Geometry: final body of the model. Coordinates: model frame, mm. A direction names the side the tool comes from. Coordinates: 2 decimals unless noted, no trailing zeros. Order: outer loops, then holes, each group sorted by start corner. A loop starts at its lowest first (then second) coordinate and runs counter-clockwise, first axis right, second up. Notation, with made-up numbers: M -4.75,36 L 12.25,36 A31 cw 12.25,70 Z; hole C 35,3 d6. An arc over 180 degrees is marked long. Use CSV: the item, a comma, the result in double quotes. Start each with the question number.
Q1. Section query C-C, the plane z = 1.6. Output: boundary loops of the cut face in (x, y), and give its area (3 significant figures).
Q2. First-contact query: P1, Ø1, axis at y = -1.5, z = 0.5, coming from the +X side. Flat tip, straight axial feed; report the tip coordinate or a pass-through.
Q3. Access query for faces 3 (the face through (-1, 2, 1.785)), 4 (the face through (2.5, 1.917, 0.859)). Directions: +Z, -Z, +X, -X, +Y, -Y. A direction counts if a zero-diameter tool reaches every point of the face in a straight line with its end or side. Return the directions, or none.
Q4. Section query D-D, the plane z = 0.5. Output: boundary loops of the cut face in (x, y), and give its area (3 significant figures).
Q5. Ray query, probe 1 along Y at (x, z) = (0, 1.55); probe 2 along X at (y, z) = (0, 0.9). Return the intervals inside material, ascending.
Q6. Mould query, pull axis X, two halves, no side actions, for faces 1 (the face through (-2.604, -0.82, 1.695)), 2 (the face through (0.748, 0.976, 1.122)). Classes: +X half, -X half, draft (parallel to the pull), parting line (faces both ways), or undercut.
Autodesk Inventor part; units mm, degrees
ref_plane "YZ Plane" through (0, 0, 0) normal (1, 0, 0) x (0, 1, 0)
ref_plane "XZ Plane" through (0, 0, 0) normal (0, 1, 0) x (-1, 0, 0)
ref_plane "XY Plane" through (0, 0, 0) normal (0, 0, 1) x (1, 0, 0)
sketch "Sketch2" plane through (0, 0, 0) normal (0, 1, 0) x (-1, 0, 0)
  line L0 (0, 0) -> (0, 2.27)
  line L1 (0, 0) -> (3.15, 0)
  line L2 (3.15, 0) -> (3.15, 1.5)
  line L3 (3.15, 1.5) -> (2.73, 1.5)
  line L4 (2.73, 1.5) -> (2.73, 1.885)
  line L5 (2.73, 1.885) -> (2.4607, 1.885)
  line L6 (2.11, 2.0775) -> (2.11, 2.27)
  line L7 (2.11, 2.27) -> (0, 2.27)
  line L8 (2.11, 2.0775) -> (1.9411, 1.785)
  line L9 (1.9411, 1.785) -> (2.403, 1.785)
  line L10 (2.403, 1.785) -> (2.4607, 1.885)
  dimension "d0" = 1.5
  dimension "d1" = 0.77
  dimension "d2" = 4.22
  dimension "d3" = 6.3
  dimension "d17" = 0.385
  dimension "d18" = 5.46
  dimension "d19" = 0.1925
  dimension "d20" = 30
  dimension "d21" = 0.1
  dimension "d23" = 0.4
revolve "Obrót1" add sketch "Sketch2" angle 360 about axis through (0, 0, 0) along (0, 0, 1)
hole "Otwór1" at (0, 0, 2.27) direction (0, 0, -1) diameter 2.459 end through all
chamfer "Faza1" distance 0.2 angle 45 3 edges at (0, 1.2295, 0) (3.15, 0, 0) (0, 1.2295, 2.27)
equation "\"d14\" = C1"
equation "\"d0\" = T_"
equation "\"d1\" = A_"
equation "\"d2\" = C_"
equation "\"d3\" = E_"
equation "\"d17\" = 0.5 * A_"
equation "\"d19\" = 0.25 * A_"
equation "\"A_\" = 0.77"
equation "\"C_\" = 4.22"
equation "\"E_\" = 6.3"
equation "\"T_\" = 1.5"
equation "\"K_\" = 0.2"
equation "\"C1\" = 0.2"
equation "\"Min_Dist\" = 4.8"
equation "\"H_Size\" = 4.25"
equation "\"Min_Thick\" = 0.8"
equation "\"NND\" = 3"
equation "\"Height\" = 2.27"
properties part number "S-M3-0 ZI" material "Stal, węglowa"
Responses:
1,outline,"C 0,0 d5.46; hole C 0,0 d2.46"
1,area,"18.7 mm²"
2,P1,"stops at x = 2.99"
3,face 3,"none"
3,face 4,"+Z, -Z"
4,outline,"C 0,0 d6.3; hole C 0,0 d2.46"
4,area,"26.4 mm²"
5,probe 1,"y = -2.73 to -1.23, 1.23 to 2.73"
5,probe 2,"x = -3.15 to -1.23, 1.23 to 3.15"
6,face 1,"parting line"
6,face 2,"undercut"
